Autodesk Inventor part; units mm, degrees
ref_plane "YZ Plane" through (0, 0, 0) normal (1, 0, 0) x (0, 1, 0)
ref_plane "XZ Plane" through (0, 0, 0) normal (0, 1, 0) x (-1, 0, 0)
ref_plane "XY Plane" through (0, 0, 0) normal (0, 0, 1) x (1, 0, 0)
sketch "Sketch1" plane through (0, 0, 0) normal (0, 0, 1) x (1, 0, 0)
  line L0 (-12.5, -19.75) -> (12.5, -19.75)
  line L1 (19.75, -12.5) -> (19.75, 12.5)
  line L2 (12.5, 19.75) -> (-12.5, 19.75)
  line L3 (-19.75, 12.5) -> (-19.75, -12.5)
  line L4 (19.75, 19.75) -> (19.75, 19.75)
  line L5 (19.75, 19.75) -> (19.75, 19.75)
  line L6 (19.75, -12.5) -> (19.75, -12.5)
  line L7 (-12.5, -19.75) -> (-19.75, -12.5)
  line L8 (-19.75, 12.5) -> (-12.5, 19.75)
  line L9 (12.5, 19.75) -> (19.75, 12.5)
  line L10 (19.75, -12.5) -> (12.5, -19.75)
  line L11 (-19.75, 0) -> (19.75, 0) construction
  circle A0 centre (0, 0) radius 10
  point P0 (19.75, 19.75)
  point P1 (19.75, -19.75)
  point P2 (-19.75, 19.75)
  dimension "d33" = 39.5
  dimension "d34" = 39.5
  dimension "d35" = 20
extrude "Extrusion7" add sketch "Sketch1" along normal blind 100
sketch "Sketch8" plane through (0, 0, 100) normal (0, 0, 1) x (1, 0, 0)
  circle A0 centre (0, 0) radius 13.75
  dimension "d38" = 27.5
extrude "Extrusion8" cut sketch "Sketch8" against normal blind 100
sketch "Sketch10" plane through (0, 0, 0) normal (0, 0, -1) x (-1, 0, 0)
  circle A0 centre (0, 0) radius 17
  dimension "d44" = 34
extrude "Extrusion10" cut sketch "Sketch10" against normal blind 25
sketch "Sketch11" plane through (0, 0, 100) normal (0, 0, 1) x (1, 0, 0)
  circle A0 centre (0, 0) radius 16.75
  line L0 (39.1509, 23.8646) -> (-32.83, 23.8646)
  line L1 (-32.83, 23.8646) -> (-32.83, -25.2836)
  line L2 (-32.83, -25.2836) -> (39.1509, -25.2836)
  line L3 (39.1509, -25.2836) -> (39.1509, 23.8646)
  dimension "d47" = 33.5
extrude "Extrusion11" cut sketch "Sketch11" against normal blind 15
sketch "Sketch12" plane through (12.5, -19.75, 85) normal (0.7071, -0.7071, 0) x (-0.7071, -0.7071, 0)
  line L0 (-10.8765, 85) -> (0.6235, 85)
  line L1 (0.6235, 85) -> (0.6235, -33.4393)
  line L2 (0.6235, -33.4393) -> (-10.8765, -33.4393)
  line L3 (-10.8765, -33.4393) -> (-10.8765, 85)
  line L4 (-5.1265, 85) -> (-5.1265, -33.4393) construction
  line L5 (0, 85) -> (-10.253, 85)
  point P0 (-5.1265, 85)
  dimension "d50" = 11.5
extrude "Extrusion12" cut sketch "Sketch12" against normal blind 20
fillet "Fillet1" radius 2 1 edges at (-12.0208, 12.0208, 0)
properties part number "conduit_endcap" material "UHMW, Black"
Here's how the part is built. I have some questions about the finished solid (model axes, mm). A direction names the side the tool comes from. Coordinates: 2 decimals unless noted, no trailing zeros. Order: outer loops, then holes, each group sorted by start corner. A loop starts at its lowest first (then second) coordinate and runs counter-clockwise, first axis right, second up. Notation, with made-up numbers: M 34,-34.75 L 39,-34.75 A15 cw 39,-21.75 Z; hole C 71,-24 d1. An arc over 180 degrees is marked long. Answer as a JSON object with one key per item and string values. Group by question number.
(1) I need wall thicknesses on probe 1 along Y at (x, z) = (0, 53.5); probe 2 along X at (y, z) = (0, 16.25). Which ranges of each line are inside material? Lowest first, please.
(2) If we mould it in two halves opening along X, with no side actions, what happens to faces 6 (the face through (16.37, -8.24, 50.7)), 7 (the face through (-11.37, 12.3, 92.6)), 8 (the face through (-19.75, 0, 42)), 9 (the face through (-6, 13, 25))? For each: released by +X, released by -X, zero draft, split by the parting line, or undercut.
(3) Suppose I cut it at C-C, the plane z = 36.5. Please give me the cut outline in (x, y).
(4) Suppose I cut it at A-A, the plane x = 0. Please give me the cut outline in (y, z), then the cut area to 3 significant figures.
(5) Which directions (+Z, -Z, +X, -X, +Y, -Y) give clear straight access to the entire face, cutting with the end or side of a thin tool? Please do faces 1 (the face through (-16.2, 10.3, 0)), 2 (the face through (19.75, 0, 42)), 3 (the face through (-15, 10, 85)), 4 (the face through (8.24, -16.37, 49.3)), 5 (the face through (-12.482, 11.541, 13.339)).
(6) For pin 1 (3 mm diameter, centred on y = -15.5, z = 50, fed in from -X); pin 2 (1.5 mm diameter, centred on x = -15.5, z = 14, fed in from +Y), each with a flat end and sliding along its axis, tell me the tip position at first contact or that it passes through.
Values found:
{
 "1": {"probe 1": "y = -19.75 to -13.75, 13.75 to 19.75", "probe 2": "x = -19.75 to -17, 17 to 19.75"},
 "2": {"face 6": "undercut", "face 7": "split by the parting line", "face 8": "released by -X", "face 9": "undercut"},
 "3": {"outline": "M -19.75,-12.5 L -12.5,-19.75 L 11.62,-19.75 L 4.77,-12.9 A13.75 cw long 12.9,-4.77 L 19.75,-11.62 L 19.75,12.5 L 12.5,19.75 L -12.5,19.75 L -19.75,12.5 Z"},
 "4": {"outline": "M -19.75,0 L -19,0 A2 ccw -17,2 L -17,25 L -13.75,25 L -13.75,100 L -16.75,100 L -16.75,85 L -19.75,85 Z; M 13.75,25 L 17,25 L 17,2 A2 ccw 19,0 L 19.75,0 L 19.75,85 L 16.75,85 L 16.75,100 L 13.75,100 Z", "area": "946 mm^2"},
 "5": {"face 1": "-Z, +X, -X, +Y, -Y", "face 2": "+Z, -Z, +X, +Y, -Y", "face 3": "+Z", "face 4": "+Z, -Z, +X", "face 5": "-Z"},
 "6": {"pin 1": "stops at x = -18.25", "pin 2": "stops at y = 17.5"}
}
